```python
from build123d import *

# Parameters (mm, degrees)
SKETCH_2_W          = 250
SKETCH_2_H          = 70
EXTRUDE_1_DEPTH     = 340
CUT_EXTRUDE_START   = -5
SKETCH_3_W          = 60
SKETCH_3_H          = 330
CUT_EXTRUDE_1_DEPTH = 240
SKETCH_4_W          = 50
SKETCH_4_H          = 325
CUT_EXTRUDE_2_DEPTH = 5
CUT_EXTRUDE_3_DEPTH = 5
FILLET_START        = -1
FILLET_1_DEPTH      = 342
SKETCH_6_W          = 13
SKETCH_6_H          = 4
CUT_EXTRUDE_4_DEPTH = 10


with BuildPart() as part:
    # 草圖2 → 填料-伸長1 (new body)
    with BuildSketch(Plane(origin=(0, 0, 0), x_dir=(1, 0, 0), z_dir=(0, 1, 0))):
        with Locations((90.582134355, -14.950757877)):
            Rectangle(SKETCH_2_W, SKETCH_2_H)
    extrude(amount=EXTRUDE_1_DEPTH)

    # 草圖3 → 除料-伸長1 (cut)
    with BuildSketch(Plane(origin=(215.582134355, 0, 0), x_dir=(0, 0, -1), z_dir=(1, 0, 0)).offset(CUT_EXTRUDE_START)):
        with Locations((-14.950757877, 170)):
            Rectangle(SKETCH_3_W, SKETCH_3_H)
    extrude(amount=-CUT_EXTRUDE_1_DEPTH, mode=Mode.SUBTRACT)

    # 草圖4 → 除料-伸長2 (cut)
    with BuildSketch(Plane(origin=(215.582134355, 0, 0), x_dir=(0, 0, -1), z_dir=(1, 0, 0))):
        with Locations((-14.950757877, 167.5)):
            Rectangle(SKETCH_4_W, SKETCH_4_H)
    extrude(amount=-CUT_EXTRUDE_2_DEPTH, mode=Mode.SUBTRACT)

    # 草圖5 → 除料-伸長3 (cut)
    with BuildSketch(Plane(origin=(0, 0, -20.049242123), x_dir=(-1, 0, 0), z_dir=(0, 0, -1))):
        Polygon((-210.582134355, 330), (-190.582134355, 330), (-190.582134355, 25), (29.417865645, 25), (29.417865645, 5), (-210.582134355, 5), align=None)
    extrude(amount=-CUT_EXTRUDE_3_DEPTH, mode=Mode.SUBTRACT)

    # 圓角1: read off the stored shape, not the designer's step
    # 圓角1 outline → 圓角1 (cut)
    with BuildSketch(Plane(origin=(0, 0, 0), x_dir=(1, 0, 0), z_dir=(0, 1, 0)).offset(FILLET_START)):
        with BuildLine():
            Line((215.582134355, 20.049242123), (210.582134355, 20.049242123))
            ThreePointArc((210.582134355, 20.049242123), (214.117668261, 18.584776029), (215.582134355, 15.049242123))
            Line((215.582134355, 15.049242123), (215.582134355, 20.049242123))
        make_face()
        with BuildLine():
            ThreePointArc((-34.417865645, 15.049242123), (-32.953399551, 18.584776029), (-29.417865645, 20.049242123))
            Line((-29.417865645, 20.049242123), (-34.417865645, 20.049242123))
            Line((-34.417865645, 20.049242123), (-34.417865645, 15.049242123))
        make_face()
        with BuildLine():
            Line((215.582134355, -49.950757877), (215.582134355, -44.950757877))
            ThreePointArc((215.582134355, -44.950757877), (214.117668261, -48.486291783), (210.582134355, -49.950757877))
            Line((210.582134355, -49.950757877), (215.582134355, -49.950757877))
        make_face()
        with BuildLine():
            ThreePointArc((-29.417865645, -49.950757877), (-32.953399551, -48.486291783), (-34.417865645, -44.950757877))
            Line((-34.417865645, -44.950757877), (-34.417865645, -49.950757877))
            Line((-34.417865645, -49.950757877), (-29.417865645, -49.950757877))
        make_face()
    extrude(amount=FILLET_1_DEPTH, mode=Mode.SUBTRACT)

    # 草圖6 → 除料-伸長4 (cut)
    with BuildSketch(Plane(origin=(0, 0, -20.049242123), x_dir=(-1, 0, 0), z_dir=(0, 0, -1))):
        with Locations((-56.582134355, 27)):
            Rectangle(SKETCH_6_W, SKETCH_6_H)
    extrude(amount=-CUT_EXTRUDE_4_DEPTH, mode=Mode.SUBTRACT)


solid = part.part
```
Read the model definition and answer for the solid it produces. Units are mm, in the model's axes. A direction names the side the tool comes from. Round coordinates to 2 decimals unless told otherwise and drop trailing zeros. Write each loop counter-clockwise with the first axis right and the second up, starting at its lowest first coordinate (ties: lowest second). Pieces come first, ordered by that corner, then holes. Notation, with made-up numbers: (80.25, 68.5) -> (88.25, 68.5) arc R26 ccw to (88.25, 95.5) -> close; hole circle Ø1 at (-11.75, 25.25). An arc over 180 degrees is marked (long way). Answer in a Markdown table with one row per item. Add a question column.
1) Which of the six approach directions +Z, -Z, +X, -X, +Y, -Y give full straight-line access (tool end or side, diameter ignored) to faces 1 (the face through (89, 168, 49.951)), 2 (the face through (92, 335, 15))?
2) Find section C-C, the plane z = 28. Determine the outline of the cut face in (x, y).
3) Find section B-B, the plane x = 127.5. Determine the outline of the cut face in (y, z).
4) Find section A-A, the plane y = 66.5. Determine the outline of the cut face in (x, z).
5) Given P1, Ø12, axis at y = 132.5, z = 29.5, coming from the +X side; P2, Ø1.2, axis at y = 26.5, z = -18, coming from the -X side; P3, Ø2.5, axis at y = 170.5, z = -17, coming from the +X side, each flat-ended and moving along its own axis, determine where each tip first touches the part or whether it passes through.
6) Determine the mould class of faces 3 (the face through (215.582, 207, 42)), 4 (the face through (91, 5, 12)), 5 (the face through (89, 340, 14)) for opening direction X: pulls with the +X half, pulls with the -X half, needs draft (parallel to the pull), parting line crosses it, or undercut.
7) Consider line 1 (Z direction, x = 26.5, y = 41.5); line 2 (Y direction, x = 47, z = 4.5); line 3 (X direction, y = 22.5, z = 42). Determine where each line is inside the solid, lowest interval first.
Findings below:
| question | item | result |
|---|---|---|
| 1 | face 1 | +Z, +X, -X, +Y, -Y |
| 1 | face 2 | none |
| 2 | outline | (-34.42, 0) -> (215.58, 0) -> (215.58, 5) -> (-29.42, 5) -> (-29.42, 335) -> (210.58, 335) -> (210.58, 330) -> (215.58, 330) -> (215.58, 340) -> (-34.42, 340) -> close |
| 3 | outline | (0, -20.05) -> (5, -20.05) -> (5, 44.95) -> (335, 44.95) -> (335, -15.05) -> (25, -15.05) -> (25, -20.05) -> (340, -20.05) -> (340, 49.95) -> (0, 49.95) -> close |
| 4 | outline | (-34.42, -15.05) arc R5 ccw to (-29.42, -20.05) -> (190.58, -20.05) -> (190.58, -15.05) -> (-29.42, -15.05) -> (-29.42, 44.95) -> (210.58, 44.95) -> (210.58, 39.95) -> (215.58, 39.95) -> (215.58, 44.95) arc R5 ccw to (210.58, 49.95) -> (-29.42, 49.95) arc R5 ccw to (-34.42, 44.95) -> close; (210.58, -20.05) arc R5 ccw to (215.58, -15.05) -> (215.58, -10.05) -> (210.58, -10.05) -> close |
| 5 | P1 | x = -29.42 |
| 5 | P2 | x = -33.83 |
| 5 | P3 | x = 215.53 |
| 6 | face 3 | pulls with the +X half |
| 6 | face 4 | undercut |
| 6 | face 5 | needs draft |
| 7 | line 1 | -20.05 to -15.05, 44.95 to 49.95 |
| 7 | line 2 | 0 to 5, 335 to 340 |
| 7 | line 3 | -34.42 to -29.42, 210.58 to 215.58 |
